Check sheet for the modelled part. Datum: model origin and axes. Units: mm. Face numbers are marked on the shaded views. A direction names the side the tool comes from. Round coordinates to 2 decimals unless told otherwise and drop trailing zeros. Loops run counter-clockwise (first coordinate to the right, second up) from the corner with the lowest first, then second, coordinate; pieces in that order, holes last. Notation, with made-up numbers: (49.25, 10) - (69.25, 10) arc R23 cw to (69.25, 33) - close; hole circle Ø6 at (-32.5, 0). An arc over 180 degrees is marked (long way). Answer in a Markdown table with one row per item. Add a question column.
(1) Gauge pin test, flat ends, axial feed: pin 1 (0.9 mm diameter, centred on x = 1, z = 3, fed in from +Y); pin 2 (0.7 mm diameter, centred on y = -0.5, z = 1.5, fed in from -X); pin 3 (3 mm diameter, centred on y = -1.5, z = 5.5, fed in from -X); pin 4 (1.9 mm diameter, centred on x = -1, y = 5, fed in from +Z). Record the tip position at first contact, or that the pin passes through.
(2) Cross-section at C-C on x = -1.5. Enter the section's corners in (y, z).
(3) Mould release check, pull along Y, two halves, no side actions. Record for the marked faces 6, 7 and 8: +Y half, -Y half, draft (parallel to the pull), parting line (faces both ways), or undercut.
(4) Access from +Z, -Z, +X, -X, +Y, -Y to the whole of each face (thin tool, end or side, straight path). Record for the marked faces 1, 2, 3, 4 and 5.
(5) Cross-section at D-D on y = -1.27. Enter the section's corners in (x, z).
(6) Thickness scan on line 1 along Y through (x, z) = (0.5, 2.25); line 2 along Z through (x, y) = (-4.5, -2.5); line 3 along X through (y, z) = (2, 1). Record the ranges inside material, lowest first.
(7) Cross-section at B-B on y = 1.27. Enter the section's corners in (x, z), then the cut area to 3 significant figures.
(8) Cross-section at A-A on z = 2.25. Enter the section's corners in (x, y), then the cut area to 3 significant figures.
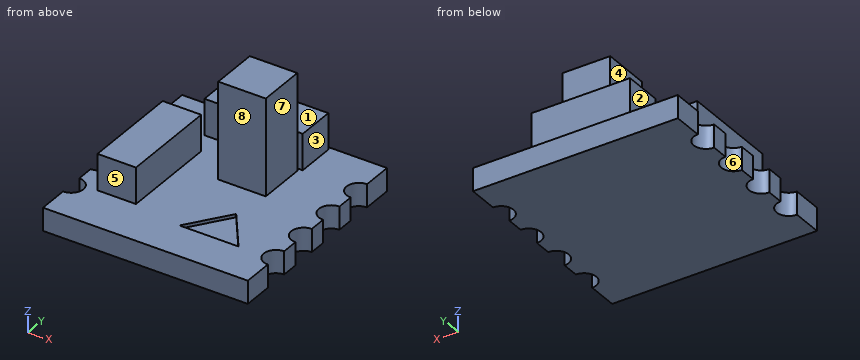
from build123d import *

# Parameters (mm, degrees)
SKETCH1_W               = 12.5
SKETCH1_H               = 12.8
BOSS_EXTRUDE1_DEPTH     = 0.7
CUT_EXTRUDE1_DEPTH      = 9.972875793
CUT_EXTRUDE1_DEPTH_BACK = 9.972875793
SKETCH2_R               = 0.75
SKETCH3_W               = 6
SKETCH3_H               = 2.35
SKETCH3_W_2             = 2.35
SKETCH3_H_2             = 6
BOSS_EXTRUDE2_DEPTH     = 2.2
SKETCH4_W               = 2.9
SKETCH4_H               = 2.9
BOSS_EXTRUDE3_DEPTH     = 5.9
CUT_EXTRUDE2_DEPTH      = 0.2


with BuildPart() as part:
    # Sketch1 → Boss-Extrude1 (new, symmetric)
    with BuildSketch(Plane.XY):
        Rectangle(SKETCH1_W, SKETCH1_H)
    extrude(amount=BOSS_EXTRUDE1_DEPTH, both=True)

    # Sketch2 → Cut-Extrude1 (cut, two sides: drawn at the far end of the back side and taken through both)
    with BuildSketch(Plane.XY.offset(-CUT_EXTRUDE1_DEPTH_BACK)):
        with Locations((-6.25, 1.27)):
            Circle(SKETCH2_R)
        with Locations((-6.25, 3.81)):
            Circle(SKETCH2_R)
        with Locations((-6.25, -1.27)):
            Circle(SKETCH2_R)
        with Locations((-6.25, -3.81)):
            Circle(SKETCH2_R)
        with Locations((6.25, -3.81)):
            Circle(SKETCH2_R)
        with Locations((6.25, -1.27)):
            Circle(SKETCH2_R)
        with Locations((6.25, 3.81)):
            Circle(SKETCH2_R)
        with Locations((6.25, 1.27)):
            Circle(SKETCH2_R)
    extrude(amount=CUT_EXTRUDE1_DEPTH + CUT_EXTRUDE1_DEPTH_BACK, mode=Mode.SUBTRACT)

    # Sketch3 → Boss-Extrude2 (add)
    with BuildSketch(Plane.XY.offset(0.7)):
        with Locations((-0.2, 5.025)):
            Rectangle(SKETCH3_W, SKETCH3_H)
        with Locations((-3.675, -0.5)):
            Rectangle(SKETCH3_W_2, SKETCH3_H_2)
    extrude(amount=BOSS_EXTRUDE2_DEPTH)

    # Sketch4 → Boss-Extrude3 (add)
    with BuildSketch(Plane.XY.offset(0.7)):
        with Locations((1.15, 2.2)):
            Rectangle(SKETCH4_W, SKETCH4_H)
    extrude(amount=BOSS_EXTRUDE3_DEPTH)

    # Sketch6 → Cut-Extrude2 (cut)
    with BuildSketch(Plane.XY.offset(0.7)):
        Polygon((2.26536139, -3.964970683), (2.26536139, -1.464970683), (0.46536139, -3.964970683), align=None)
        Polygon((4.06536139, -3.964970683), (2.26536139, -1.464970683), (2.26536139, -3.964970683), align=None)
    extrude(amount=-CUT_EXTRUDE2_DEPTH, mode=Mode.SUBTRACT)


solid = part.part
Answers:
| question | item | result |
|---|---|---|
| 1 | pin 1 | stops at y = 6.2 |
| 1 | pin 2 | stops at x = -4.85 |
| 1 | pin 3 | passes through |
| 1 | pin 4 | stops at z = 2.9 |
| 2 | outline | (-6.4, -0.7) - (6.4, -0.7) - (6.4, 0.7) - (6.2, 0.7) - (6.2, 2.9) - (3.85, 2.9) - (3.85, 0.7) - (-6.4, 0.7) - close |
| 3 | face 6 | undercut |
| 3 | face 7 | draft |
| 3 | face 8 | -Y half |
| 4 | face 1 | +Z, +X, -X, +Y |
| 4 | face 2 | +Z, -X, +Y |
| 4 | face 3 | +Z, +X, +Y, -Y |
| 4 | face 4 | +Z, -Y |
| 4 | face 5 | +Z, +X, -X, -Y |
| 5 | outline | (-5.5, -0.7) - (5.5, -0.7) - (5.5, 0.7) - (-2.5, 0.7) - (-2.5, 2.9) - (-4.85, 2.9) - (-4.85, 0.7) - (-5.5, 0.7) - close |
| 6 | line 1 | y = 0.75 to 3.65, 3.85 to 6.2 |
| 6 | line 2 | z = -0.7 to 2.9 |
| 6 | line 3 | x = -4.85 to -2.5, -0.3 to 2.6 |
| 7 | outline | (-5.5, -0.7) - (5.5, -0.7) - (5.5, 0.7) - (2.6, 0.7) - (2.6, 6.6) - (-0.3, 6.6) - (-0.3, 0.7) - (-2.5, 0.7) - (-2.5, 2.9) - (-4.85, 2.9) - (-4.85, 0.7) - (-5.5, 0.7) - close |
| 7 | area | 37.7 mm^2 |
| 8 | outline | (-4.85, -3.5) - (-2.5, -3.5) - (-2.5, 2.5) - (-4.85, 2.5) - close; (-3.2, 3.85) - (2.8, 3.85) - (2.8, 6.2) - (-3.2, 6.2) - close; (-0.3, 0.75) - (2.6, 0.75) - (2.6, 3.65) - (-0.3, 3.65) - close |
| 8 | area | 36.6 mm^2 |
